Verification items for the finished model (mm, model axes). Face numbers are marked on the shaded views. Coordinates: 2 decimals unless noted, no trailing zeros. Order: outer loops, then holes, each group sorted by start corner. A loop starts at its lowest first (then second) coordinate and runs counter-clockwise, first axis right, second up.
Q1. Cross-section at A-A, the plane z = 0. Record the boundary of the cut face in (x, y), and give its area (3 significant figures).
Q2. Cross-section at B-B, the plane y = -1.25. Record the boundary of the cut face in (x, z), and give its area (3 significant figures).
Q3. Cross-section at D-D, the plane z = -2.25. Record the boundary of the cut face in (x, y), and give its area (3 significant figures).
Q4. Depth check by flat-ended pin: P1, Ø2, axis at x = 3, y = -0.5, coming from the +Z side; P2, Ø2, axis at x = -1, y = 1, coming from the +Z side; P3, Ø1.5, axis at x = 1.5, y = -0.5, coming from the -Z side. Enter the tip coordinate at first touch or a pass-through.
Q5. Draft check along X on the marked faces 1 and 2. Enter one of: pulls with the +X half, pulls with the -X half, needs draft (parallel to the pull), parting line crosses it, or undercut.
Q6. Cross-section at C-C, the plane x = 3. Record the boundary of the cut face in (y, z), and give its area (3 significant figures).
Q7. Thickness scan on line 1 (X direction, y = 0.7, z = 0); line 2 (X direction, y = 1.5, z = -0.5); line 3 (Z direction, x = 0.75, y = -1.75). Record the ranges inside material, lowest first.
from build123d import *

# Parameters (mm, degrees)
CUT_EXTRUDE_1_DEPTH = 5
SKETCH_4_R          = 1.5
CUT_EXTRUDE_2_DEPTH = 10
CHAMFER_1_SIZE      = 0.5


with BuildPart() as part:
    # 草图1 → 旋转1 (revolve)
    with BuildSketch(Plane.XY):
        with BuildLine():
            Line((0, 4), (0, -4))
            ThreePointArc((0, -4), (4, 0), (0, 4))
        make_face()
    revolve(axis=Axis((0, 4, 0), (0, -1, 0)))

    # 草图3 → 切除-拉伸1 (cut, symmetric)
    with BuildSketch(Plane(origin=(0, 0, 0), x_dir=(0, 0, -1), z_dir=(1, 0, 0))):
        with BuildLine():
            Line((-2.645751311, 3), (2.645751311, 3))
            ThreePointArc((2.645751311, 3), (0, 4), (-2.645751311, 3))
        make_face()
        with BuildLine():
            Line((-2.645751311, -3), (2.645751311, -3))
            ThreePointArc((2.645751311, -3), (0, -4), (-2.645751311, -3))
        make_face()
    extrude(amount=CUT_EXTRUDE_1_DEPTH, both=True, mode=Mode.SUBTRACT)

    # 草图4 → 切除-拉伸2 (cut)
    with BuildSketch(Plane.XZ.offset(3)):
        with Locations(Location((0, 0, 0), (0, 0, 270))):
            Circle(SKETCH_4_R)
    extrude(amount=-CUT_EXTRUDE_2_DEPTH, mode=Mode.SUBTRACT)

    # 倒角1
    chamfer_1_edges = [part.edges().sort_by_distance(p)[0] for p in [
        (0, 3, 1.5),
        (0, -3, 1.5),
    ]]
    chamfer(chamfer_1_edges, length=CHAMFER_1_SIZE)


solid = part.part
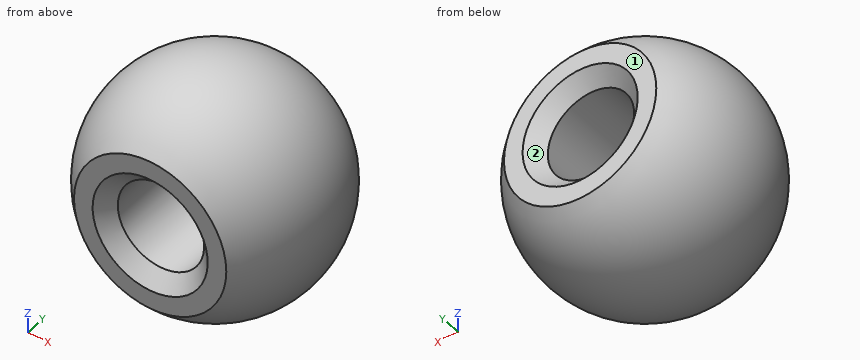
Check values:
1. outline: (-2.65, -3) - (-2, -3) - (-1.5, -2.5) - (-1.5, 2.5) - (-2, 3) - (-2.65, 3) arc R4 ccw to start; (1.5, -2.5) - (2, -3) - (2.65, -3) arc R4 ccw to (2.65, 3) - (2, 3) - (1.5, 2.5) - close
1. area: 24.5 mm2
2. outline: circle Ø7.6 at (0, 0); hole circle Ø3 at (0, 0)
2. area: 38.3 mm2
3. outline: (-1.39, -3) - (1.39, -3) arc R3.31 ccw to (1.39, 3) - (-1.39, 3) arc R3.31 ccw to start
3. area: 33.2 mm2
4. P1: stops at z = 3.44
4. P2: stops at z = 3.98
4. P3: stops at z = -3.91
5. face 1: needs draft
5. face 2: undercut
6. outline: circle Ø5.29 at (0, 0)
6. area: 22.0 mm2
7. line 1: x = -3.94 to -1.5, 1.5 to 3.94
7. line 2: x = -3.67 to -1.41, 1.41 to 3.67
7. line 3: z = -3.52 to -1.3, 1.3 to 3.52
